Verification items for the finished model (mm, model axes). A direction names the side the tool comes from. Round coordinates to 2 decimals unless told otherwise and drop trailing zeros. Order: outer loops, then holes, each group sorted by start corner. A loop starts at its lowest first (then second) coordinate and runs counter-clockwise, first axis right, second up. Notation, with made-up numbers: (-7.75, 35) -> (18.25, 35) arc R19 ccw to (18.25, 62) -> close; hole circle Ø4 at (7, 87). An arc over 180 degrees is marked (long way). Put each result on its own line as item: value.
Autodesk Inventor part; units mm, degrees
ref_plane "YZ Plane" through (0, 0, 0) normal (1, 0, 0) x (0, 1, 0)
ref_plane "XZ Plane" through (0, 0, 0) normal (0, 1, 0) x (-1, 0, 0)
ref_plane "XY Plane" through (0, 0, 0) normal (0, 0, 1) x (1, 0, 0)
sketch "Эскиз1" plane through (0, 0, 0) normal (0, 0, 1) x (1, 0, 0)
  line L0 (0, 0) -> (0, 5)
  line L1 (0, 5) -> (10, 5)
  line L2 (10, 5) -> (10, 4)
  line L3 (10, 4) -> (13, 4)
  line L4 (13, 4) -> (13, 6.15)
  line L5 (13, 6.15) -> (30, 7)
  line L6 (30, 7) -> (67, 7)
  line L7 (67, 7) -> (67, 10)
  line L8 (67, 10) -> (70, 10)
  line L9 (70, 10) -> (70, 0)
  line L10 (0, 0) -> (70, 0)
  dimension "d0" = 10
  dimension "d1" = 12.3
  dimension "d2" = 14
  dimension "d3" = 10
  dimension "d4" = 3
  dimension "d5" = 20
  dimension "d6" = 8
  dimension "d7" = 60
  dimension "d8" = 3
  dimension "d9" = 20
revolve "Вращение1" add sketch "Эскиз1" angle 360 about axis through (0, 0, 0) along (1, 0, 0)
thread "Резьба1"
chamfer "Фаска1" distance 1 angle 45 2 edges at (0, -5, 0) (10, -5, 0)
fillet "Сопряжение1" radius 0.5 2 edges at (10, -4.0001, 0) (10, -4, 0)
fillet "Сопряжение2" radius 1 1 edges at (13, -4, 0)
properties part number "Палец_ребрышко"
Item 1: Sectioned sample at D-D, the plane x = 11. Record the boundary of the cut face in (y, z), then the cut area to 3 significant figures.
Geometry check:
outline: circle Ø8 at (0, 0)
area: 50.3 mm2
Item 2: Sectioned sample at A-A, the plane z = 0. Record the boundary of the cut face in (x, y), then the cut area to 3 significant figures.
Geometry check:
outline: (0, -4) -> (1, -5) -> (9, -5) -> (9.85, -4.15) arc R0.5 cw to (10.21, -4) -> (12, -4) arc R1 cw to (13, -5) -> (13, -6.15) -> (30, -7) -> (67, -7) -> (67, -10) -> (70, -10) -> (70, 10) -> (67, 10) -> (67, 7) -> (30, 7) -> (13, 6.15) -> (13, 5) arc R1 cw to (12, 4) -> (10.21, 4) arc R0.5 cw to (9.85, 4.15) -> (9, 5) -> (1, 5) -> (0, 4) -> close
area: 924 mm2
Item 3: Tool access check on faces 1 (the face through (0, 0, 0)), 2 (the face through (67, 2, 7)). Record the directions out of +Z, -Z, +X, -X, +Y, -Y that give a thin tool (end or side, any length) a straight path to the whole face; none if there is none.
Geometry check:
face 1: +Z, -Z, -X, +Y, -Y
face 2: -X
Item 4: Material ranges on line 1 along X through (y, z) = (2, -5.75); line 2 along X through (y, z) = (8, 5); line 3 along X through (y, z) = (0, -4.75), recorded low to high.
Geometry check:
line 1: 13 to 70
line 2: 67 to 70
line 3: 0.75 to 9.25, 12.97 to 70
Item 5: Sectioned sample at C-C, the plane x = 62.5. Record the boundary of the cut face in (y, z), then the cut area to 3 significant figures.
Geometry check:
outline: circle Ø14 at (0, 0)
area: 154 mm2
Item 6: Depth check by flat-ended pin: pin 1 Ø3.5 at (y, z) = (2.5, 1) entering from -X; pin 2 Ø8 at (x, y) = (54, -0.5) entering from +Z; pin 3 Ø12 at (x, z) = (46.5, -1.5) entering from +Y; pin 4 Ø12 at (x, z) = (60, 4) entering from -Y. Enter the tip coordinate at first touch or a pass-through.
Geometry check:
pin 1: x = 0
pin 2: z = 7
pin 3: y = 7
pin 4: y = -7
Item 7: Release check for a two-part mould opening along X. For faces 3 (the face through (68.52, -2.17, -9.76)), 4 (the face through (21.619, -1.427, -6.424)), 5 (the face through (11.116, -0.867, -3.905)), 6 (the face through (70, 0, 0)) record: pulls with the +X half, pulls with the -X half, needs draft (parallel to the pull), parting line crosses it, or undercut.
Geometry check:
face 3: needs draft
face 4: pulls with the -X half
face 5: undercut
face 6: pulls with the +X half
